The model under review builds one solid part; all positions refer to its coordinate system, in mm. A direction names the side the tool comes from. Round coordinates to 2 decimals unless told otherwise and drop trailing zeros. Order: outer loops, then holes, each group sorted by start corner. A loop starts at its lowest first (then second) coordinate and runs counter-clockwise, first axis right, second up.
from build123d import *

# Parameters (mm, degrees)
SKETCH_1_W          = 50
SKETCH_1_H          = 60
EXTRUDE_1_DEPTH     = 10.6
EXTRUDE_2_DEPTH     = 3
EXTRUDE_START       = -18.2
EXTRUDE_3_DEPTH     = 3
SWEEP_START         = -7.6
SWEEP_1_DEPTH       = 15.2
SKETCH_4_R          = 1.65
CUT_EXTRUDE_1_DEPTH = 3


# Read off the part's stored shape, not the designer's step: the sweep step
with BuildPart() as part:
    # Sketch 1 → Extrude 1 (new, symmetric)
    with BuildSketch(Plane.XY):
        Rectangle(SKETCH_1_W, SKETCH_1_H)
    extrude(amount=EXTRUDE_1_DEPTH, both=True)

    # Sketch 2 → Extrude 2 (add)
    with BuildSketch(Plane.XY.offset(10.6)):
        Polygon((-25, 30), (25, 30), (25, 40.627828084), align=None)
    extrude(amount=-EXTRUDE_2_DEPTH)

    # Sketch 2_2 → Extrude 3 (add)
    with BuildSketch(Plane.XY.offset(10.6).offset(EXTRUDE_START)):
        Polygon((-25, 30), (25, 30), (25, 40.627828084), align=None)
    extrude(amount=-EXTRUDE_3_DEPTH)

    # Sweep 1 outline → Sweep 1 (cut)
    with BuildSketch(Plane.XY.offset(SWEEP_START)):
        Polygon((-25, 30), (-25, 14), (25, 24.627828084), (25, 30), align=None)
    extrude(amount=SWEEP_1_DEPTH, mode=Mode.SUBTRACT)

    # Sketch 4 → Cut-Extrude 1 (cut)
    with BuildSketch(Plane.XY.offset(-7.6)):
        with Locations((-4.562952015, 26.011583112)):
            Circle(SKETCH_4_R)
        with Locations((5.218523993, 28.09070002)):
            Circle(SKETCH_4_R)
        with Locations((15, 30.169816928)):
            Circle(SKETCH_4_R)
    cut_extrude_1 = extrude(amount=-CUT_EXTRUDE_1_DEPTH, mode=Mode.SUBTRACT)

    # Mirror 1: Cut-Extrude 1 across plane
    add(cut_extrude_1.mirror(Plane.XY), mode=Mode.SUBTRACT)


solid = part.part
(1) We need section C-C (z = 0.5). Give the boundary of the cut face in (x, y), and give its area (3 significant figures).
(2) To check wall thickness, follow L1, parallel to Z at x = 23, y = 35; L2, parallel to Y at x = 15, z = 8.75; L3, parallel to Y at x = -5, z = 5.5. State the ranges of each line that lie inside material, in increasing order.
(3) Clearance check with a flat-ended pin moving along its axis: P1, Ø3, axis at x = -13, z = -5.5, coming from the +Y side. State where the tip first meets the part, or that it passes through.
(4) We need section A-A (x = 15). Give the boundary of the cut face in (y, z), and give its area (3 significant figures).
(5) The part is to be moulded in two halves that separate along Y. For faces 3 (the cylindrical face through (-4.92, 24.4, 9.08)), 4 (the flat face through (0, 28, 7.6)), 5 (the flat face through (0, -30, 0)), 6 (the flat face through (-0.35, 19.24, -0.11)), say which applies: pulls with the +Y half, pulls with the -Y half, needs draft (parallel to the pull), parting line crosses it, or undercut.
(6) We need section B-B (x = 4.5). Give the boundary of the cut face in (y, z), and give its area (3 significant figures).
(7) Tool access review of faces 1 (the flat face through (-25, -7, 0)), 2 (the flat face through (0, 28, -7.6)): name each direction out of +Z, -Z, +X, -X, +Y, -Y from which nothing blocks a thin tool from reaching the whole face with its end or side.
(8) We need section D-D (x = -10). Give the boundary of the cut face in (y, z).
Verdict:
1. outline: (-25, -30) - (25, -30) - (25, 24.63) - (-25, 14) - close
1. area: 2,470 mm2
2. L1: z = -10.6 to -7.6, 7.6 to 10.6
2. L2: y = -30 to 28.52, 31.82 to 38.5
2. L3: y = -30 to 18.25
3. P1: stops at y = 16.87
4. outline: (-30, -10.6) - (28.52, -10.6) - (28.52, -7.6) - (22.5, -7.6) - (22.5, 7.6) - (28.52, 7.6) - (28.52, 10.6) - (-30, 10.6) - close; (31.82, -10.6) - (38.5, -10.6) - (38.5, -7.6) - (31.82, -7.6) - close; (31.82, 7.6) - (38.5, 7.6) - (38.5, 10.6) - (31.82, 10.6) - close
4. area: 1,190 mm2
5. face 3: undercut
5. face 4: needs draft
5. face 5: pulls with the -Y half
5. face 6: pulls with the +Y half
6. outline: (-30, -10.6) - (26.61, -10.6) - (26.61, -7.6) - (20.27, -7.6) - (20.27, 7.6) - (26.61, 7.6) - (26.61, 10.6) - (-30, 10.6) - close; (29.58, -10.6) - (36.27, -10.6) - (36.27, -7.6) - (29.58, -7.6) - close; (29.58, 7.6) - (36.27, 7.6) - (36.27, 10.6) - (29.58, 10.6) - close
6. area: 1,140 mm2
7. face 1: +Z, -Z, -X, +Y, -Y
7. face 2: -X, +Y
8. outline: (-30, -10.6) - (33.19, -10.6) - (33.19, -7.6) - (17.19, -7.6) - (17.19, 7.6) - (33.19, 7.6) - (33.19, 10.6) - (-30, 10.6) - close
